Geometry check sheet. Reference: drawing and pictorial views, mm from the part's lowest x, y, z. Round coordinates to 2 decimals unless told otherwise and drop trailing zeros. Write each loop counter-clockwise with the first axis right and the second up, starting at its lowest first coordinate (ties: lowest second). Pieces come first, ordered by that corner, then holes. Notation, with made-up numbers: (82.5, 75) -> (128.5, 75) arc R21 ccw to (128.5, 106) -> close; hole circle Ø7 at (38, -12). An arc over 180 degrees is marked (long way). Answer as a JSON object with one key per item and string values. Group by question number.
(1) Gauge pin test, flat ends, axial feed: pin 1 Ø6 at (y, z) = (2, 44.5) entering from -X; pin 2 Ø6 at (x, y) = (34, 2.5) entering from +Z; pin 3 Ø4 at (x, y) = (32, 7.5) entering from +Z. Record the tip position at first contact, or that the pin passes through.
(2) Scan lines: L1, parallel to Y at x = 11, z = 37.5; L2, parallel to Z at x = 2.5, y = 12; L3, parallel to X at y = 8, z = 79.5. Record each from-to range of solid material in increasing order. Write a range as from..to.
(3) Sectioned sample at B-B on x = 15. Record the cut outline in (y, z).
(4) Sectioned sample at D-D on y = 2.25. Record the cut outline in (x, z).
(5) Sectioned sample at C-C on z = 39.5. Record the cut outline in (x, y).
(6) Sectioned sample at A-A on y = 8.5. Record the cut outline in (x, z), and give its area (3 significant figures).
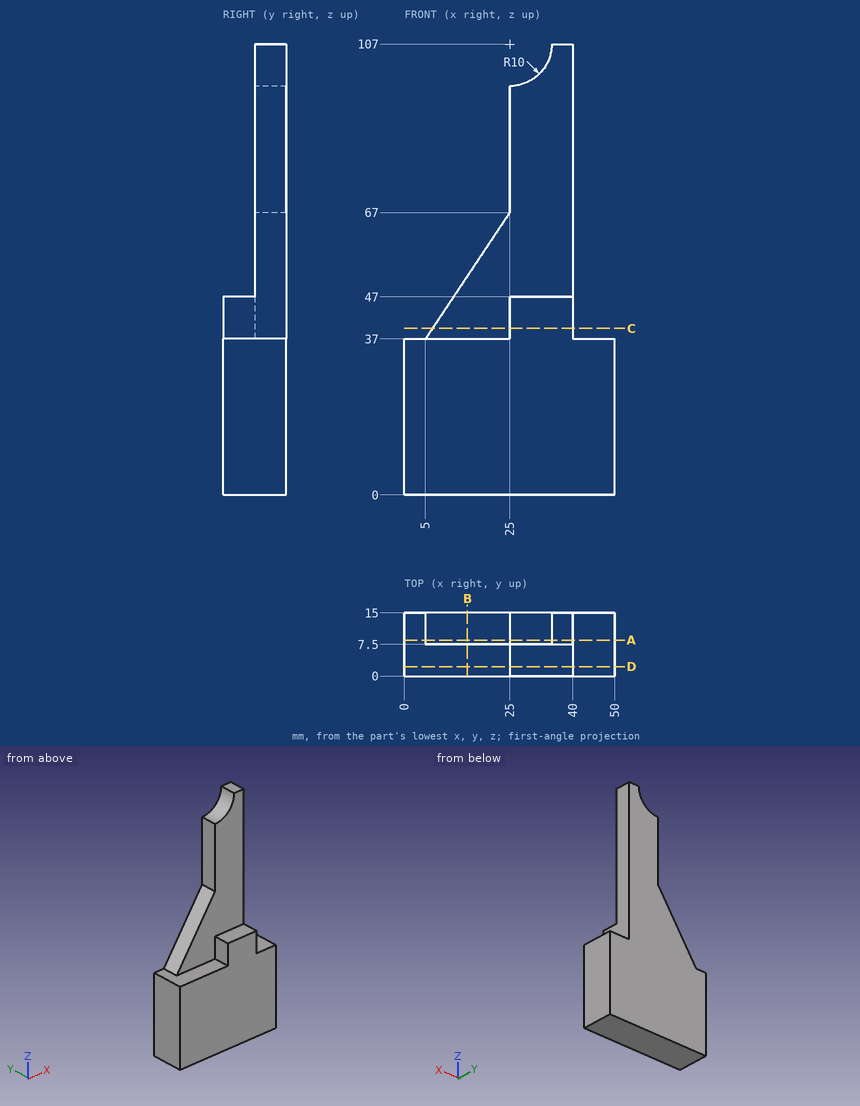
Computed values:
{
 "1": {"pin 1": "x = 25", "pin 2": "z = 47", "pin 3": "z = 102.64"},
 "2": {"L1": "7.5..15", "L2": "0..37", "L3": "25..40"},
 "3": {"outline": "(0, 0) -> (15, 0) -> (15, 52) -> (7.5, 52) -> (7.5, 37) -> (0, 37) -> close"},
 "4": {"outline": "(0, 0) -> (50, 0) -> (50, 37) -> (40, 37) -> (40, 47) -> (25, 47) -> (25, 37) -> (0, 37) -> close"},
 "5": {"outline": "(6.67, 7.5) -> (25, 7.5) -> (25, 0) -> (40, 0) -> (40, 15) -> (6.67, 15) -> close"},
 "6": {"outline": "(0, 0) -> (50, 0) -> (50, 37) -> (40, 37) -> (40, 107) -> (35, 107) arc R10 cw to (25, 97) -> (25, 67) -> (5, 37) -> (0, 37) -> close", "area": "3,120 mm2"}
}
